Source: three-view drawing plus pictorial views. Frame: mm from the lowest corner of the part. A direction names the side the tool comes from. Coordinates: 2 decimals unless noted, no trailing zeros. Order: outer loops, then holes, each group sorted by start corner. A loop starts at its lowest first (then second) coordinate and runs counter-clockwise, first axis right, second up. Notation, with made-up numbers: (26, 63) - (68, 63) arc R21 cw to (68, 100) - close; hole circle Ø8 at (65, 4). An arc over 180 degrees is marked (long way). One line per question, with ' | ' between items.
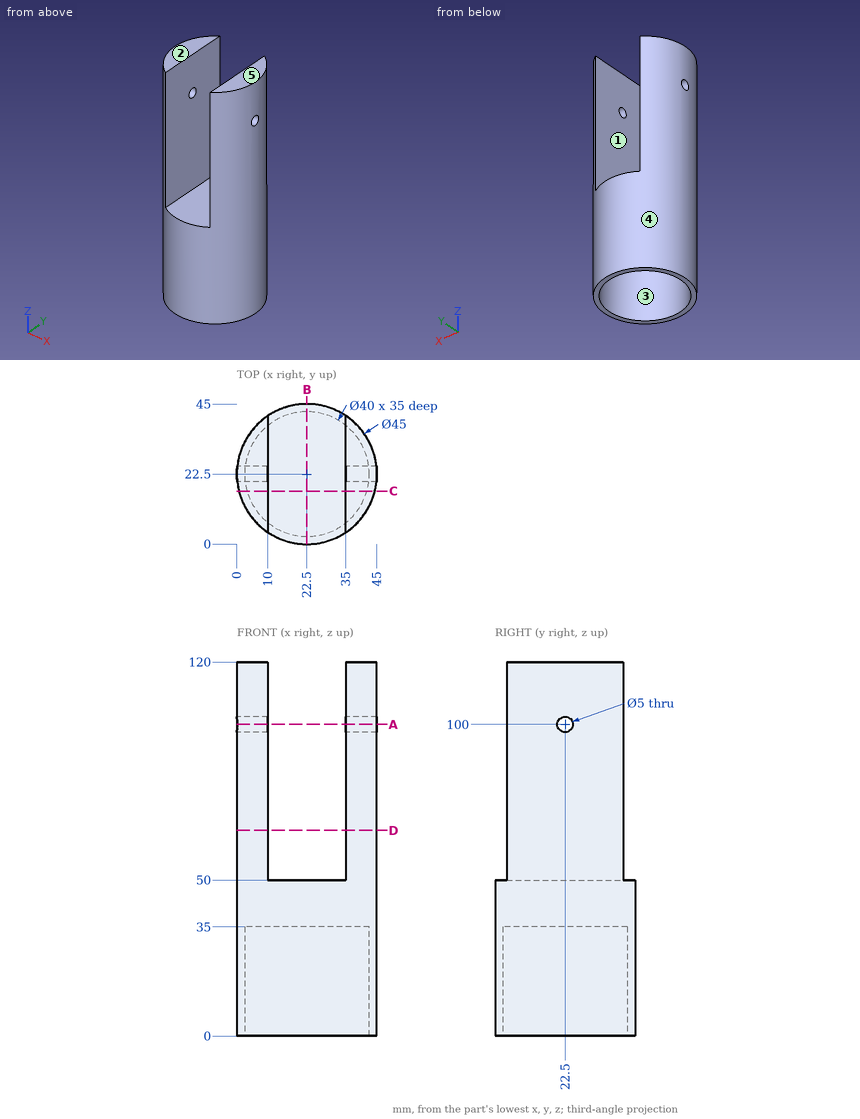
Item 1: Section A-A on z = 100. Return the cut outline in (x, y).
Data:
outline: (0.14, 20) arc R22.5 ccw to (10, 3.79) - (10, 20) - close; (0.14, 25) - (10, 25) - (10, 41.21) arc R22.5 ccw to start; (35, 3.79) arc R22.5 ccw to (44.86, 20) - (35, 20) - close; (35, 25) - (44.86, 25) arc R22.5 ccw to (35, 41.21) - close
Item 2: Section C-C on y = 17. Return the cut outline in (x, z), and give its area (3 significant figures).
Data:
outline: (0.68, 0) - (3.27, 0) - (3.27, 35) - (41.73, 35) - (41.73, 0) - (44.32, 0) - (44.32, 120) - (35, 120) - (35, 50) - (10, 50) - (10, 120) - (0.68, 120) - close | area: 2,140 mm^2
Item 3: Contact query for flat-ended pins moving along their axis: P1, Ø11, axis at y = 14.5, z = 83, coming from the -X side; P2, Ø6, axis at x = 29.5, z = 47.5, coming from the -Y side; P3, Ø1.5, axis at x = 26, z = 42.5, coming from the -Y side; P4, Ø18.5, axis at y = 17.5, z = 91, coming from the +X side. Output: stop coordinate, or through.
Data:
P1: x = 0.14 | P2: y = 0.36 | P3: y = 0.17 | P4: x = 45
Item 4: Section D-D on z = 66. Return the cut outline in (x, y), and give its area (3 significant figures).
Data:
outline: (10, 3.79) - (10, 41.21) arc R22.5 ccw to start; (35, 3.79) arc R22.5 ccw to (35, 41.21) - close | area: 526 mm^2
Item 5: Draft query along X for the marked faces 3, 4 and 5. Return one class per face: released by +X, released by -X, zero draft, split by the parting line, or undercut.
Data:
face 3: undercut | face 4: split by the parting line | face 5: zero draft
Item 6: Section B-B on x = 22.5. Return the cut outline in (y, z).
Data:
outline: (0, 0) - (2.5, 0) - (2.5, 35) - (42.5, 35) - (42.5, 0) - (45, 0) - (45, 50) - (0, 50) - close
Item 7: Ray query, line 1 (Y direction, x = 22, z = 27); line 2 (Z direction, x = 41.75, y = 22.5); line 3 (Z direction, x = 38.5, y = 28). Return the intervals inside material, ascending.
Data:
line 1: 0.01 to 2.51, 42.49 to 44.99 | line 2: 35 to 97.5, 102.5 to 120 | line 3: 35 to 120
Item 8: Access query for the marked faces 1 and 2. Directions: +Z, -Z, +X, -X, +Y, -Y. A direction counts if a zero-diameter tool reaches every point of the face in a straight line with its end or side. Return the directions, or none.
Data:
face 1: +Z, +Y, -Y | face 2: +Z, +X, -X, +Y, -Y
